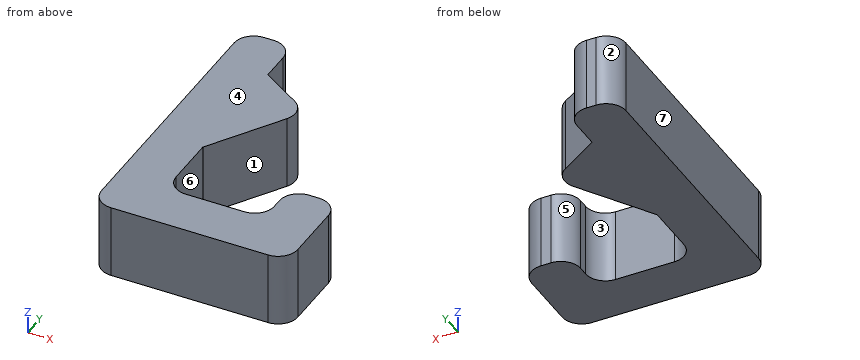
from build123d import *

# Parameters (mm, degrees)
F1_DEPTH = 7.5


with BuildPart() as f1:
    # F0 (on Top) → F1 (new body)
    with BuildSketch(Plane.XY):
        with BuildLine():
            ThreePointArc((-18, 30), (-19.414214, 29.414214), (-20, 28))
            Line((-20, 28), (-20, 2))
            ThreePointArc((-20, 2), (-19.414214, 0.585786), (-18, 0))
            Line((-18, 0), (-2, 0))
            ThreePointArc((-2, 0), (-0.585786, 0.585786), (0, 2))
            Line((0, 2), (0, 8))
            ThreePointArc((0, 8), (-0.585786, 9.414214), (-2, 10))
            Line((-2, 10), (-3, 10))
            ThreePointArc((-3, 10), (-4.414214, 9.414214), (-5, 8))
            Line((-5, 8), (-5, 7))
            ThreePointArc((-5, 7), (-5.585786, 5.585786), (-7, 5))
            Line((-7, 5), (-13, 5))
            ThreePointArc((-13, 5), (-14.414214, 5.585786), (-15, 7))
            Line((-15, 7), (-15, 12.231735))
            Line((-15, 12.231735), (-10.307771, 19.680434))
            ThreePointArc((-10.307771, 19.680434), (-10.049636, 21.189245), (-10.933998, 22.438665))
            Line((-10.933998, 22.438665), (-15, 25))
            Line((-15, 25), (-15, 28))
            ThreePointArc((-15, 28), (-15.585786, 29.414214), (-17, 30))
            Line((-17, 30), (-18, 30))
        make_face()
    extrude(amount=F1_DEPTH)


solid = f1.part
Can you work these out from the model? Positions are in its coordinate system, mm. Face numbers are marked on the shaded views. A direction names the side the tool comes from. Give positions to 0.01 mm unless a question says otherwise; leave off trailing zeros. Order: outer loops, then holes, each group sorted by start corner. A loop starts at its lowest first (then second) coordinate and runs counter-clockwise, first axis right, second up. Notation, with made-up numbers: M 89,24.25 L 128,24.25 A20 cw 128,30.25 Z; hole C 7.25,-24 d3. An arc over 180 degrees is marked long. Use a Markdown table: item, result. Add a question column.
Item 1: Will these pins go through, and if not, where does the flat tip stop? pin 1 (1.5 mm diameter, centred on x = -14.5, z = 4.5, fed in from +Y); pin 2 (2 mm diameter, centred on y = 12.5, z = 5.5, fed in from +X); pin 3 (1.1 mm diameter, centred on x = -2.5, z = 5, fed in from +Y).
Item 2: For the marked faces 5, 6 and 7, which set-ups out of +Z, -Z, +X, -X, +Y, -Y let a thin tool reach every point of the face, with its end or its side?
Item 3: We'd pull the mould along X, two halves only. Please class the marked faces 1, 2, 3 and 4: +X half, -X half, draft (parallel to the pull), parting line (faces both ways), or undercut.
Item 4: Suppose I cut it at C-C (y = 26.5). List the corners of the cut face in (x, z) for me, then the cut area to 3 significant figures.
Item 5: If I drill on L1, parallel to X at y = 8, z = 3.25; L2, parallel to X at y = 11.5, z = 0.5; L3, parallel to Y at x = -14.25, z = 3.75, over which ranges is the centre line in solid material (lowest first)? Write a range as [from, to].
Item 6: Suppose I cut it at B-B (z = 4.25). List the corners of the cut face in (x, y) for me.
Item 7: Suppose I cut it at D-D (x = -5.75). List the corners of the cut face in (y, z) for me, then the cut area to 3 significant figures.
Item 8: Suppose I cut it at A-A (x = -14). List the corners of the cut face in (y, z) for me.
Answer sheet:
| question | item | result |
|---|---|---|
| 1 | pin 1 | stops at y = 28.97 |
| 1 | pin 2 | stops at x = -14.2 |
| 1 | pin 3 | stops at y = 10 |
| 2 | face 5 | +Z, -Z, +Y |
| 2 | face 6 | +Z, -Z |
| 2 | face 7 | +Z, -Z, -X, +Y, -Y |
| 3 | face 1 | +X half |
| 3 | face 2 | -X half |
| 3 | face 3 | undercut |
| 3 | face 4 | draft |
| 4 | outline | M -20,0 L -15,0 L -15,7.5 L -20,7.5 Z |
| 4 | area | 37.5 mm² |
| 5 | L1 | x = [-20, -15], [-5, 0] |
| 5 | L2 | x = [-20, -15] |
| 5 | L3 | y = [0, 5.44], [13.42, 24.53] |
| 6 | outline | M -20,2 A2 ccw -18,0 L -2,0 A2 ccw 0,2 L 0,8 A2 ccw -2,10 L -3,10 A2 ccw -5,8 L -5,7 A2 cw -7,5 L -13,5 A2 cw -15,7 L -15,12.23 L -10.31,19.68 A2 ccw -10.93,22.44 L -15,25 L -15,28 A2 ccw -17,30 L -18,30 A2 ccw -20,28 Z |
| 7 | outline | M 0,0 L 5.44,0 L 5.44,7.5 L 0,7.5 Z |
| 7 | area | 40.8 mm² |
| 8 | outline | M 0,0 L 5.27,0 L 5.27,7.5 L 0,7.5 Z; M 13.82,0 L 24.37,0 L 24.37,7.5 L 13.82,7.5 Z |
